Read the model definition and answer for the solid it produces. Units are mm, in the model's axes. Face numbers are marked on the shaded views. A direction names the side the tool comes from. Coordinates: 2 decimals unless noted, no trailing zeros. Order: outer loops, then holes, each group sorted by start corner. A loop starts at its lowest first (then second) coordinate and runs counter-clockwise, first axis right, second up. Notation, with made-up numbers: (59, -2.75) -> (117, -2.75) arc R27 ccw to (117, 14.25) -> close; hole circle Ø5 at (-32, 11.5). An arc over 180 degrees is marked (long way). Answer in a Markdown table with one row per item.
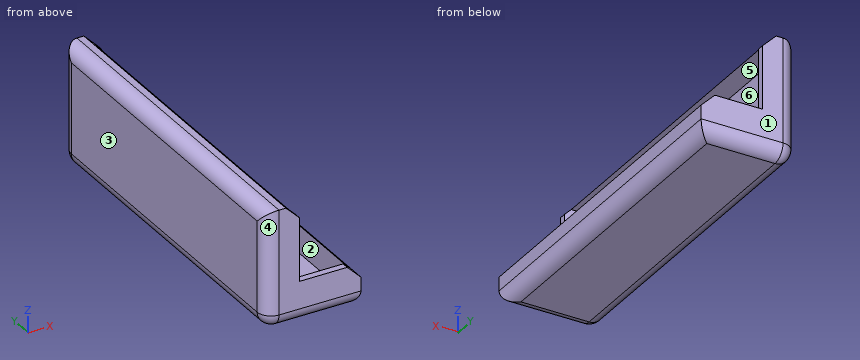
from build123d import *

# Parameters (mm, degrees)
F0_W        = 22.6290904153
F0_H        = 15.2400004526
F1_DEPTH    = 127
F2_T        = -2.54
F3_R        = 5.08
F4_T1_DEPTH = 153.1282991577


# Not quite as in the source:
# - a fillet or chamfer that OpenCascade refuses, or shapes differently, is made with other operations: its cross-section is extruded or revolved along the edge and cut away or added


with BuildPart() as f1:
    # F0 (on Front) → F1 (new body)
    with BuildSketch(Plane.XZ):
        Polygon((-22.6290904153, 0), (-22.6290904153, 15.2400004526), (-22.6290904153, 43.6418191694), (-35.3290904153, 43.6418191694), (-35.3290904153, 0), align=None)
        with Locations((-11.3145452077, 7.6200002263)):
            Rectangle(F0_W, F0_H)
    extrude(amount=F1_DEPTH)

    # F2
    f2_openings = [f1.faces().sort_by_distance(p)[0] for p in [
        (-22.62909, -63.5, 29.44091),
        (-11.314545, -63.5, 15.24),
    ]]
    offset(amount=F2_T, openings=f2_openings)

    # F3
    f3_edges = [f1.edges().sort_by_distance(p)[0] for p in [
        (-35.32909, -63.5, 43.641819),
        (0, -63.5, 0),
        (-35.32909, -63.5, 0),
        (-35.32909, 0, 21.82091),
        (-35.32909, -127, 21.82091),
        (-17.664545, -127, 0),
        (-17.664545, 0, 0),
    ]]
    fillet(f3_edges, radius=F3_R)

    # F4: chamfer of 5.08 on 2 edges, made by hand

    # F4_s2 → F4_t1 (cut)
    with BuildSketch(Plane.XZ.offset(-13.0641495789)):
        Polygon((-27.7090904153, 43.6418191694), (-22.6290904153, 38.5618191694), (-22.6290904153, 43.6418191694), align=None)
        Polygon((-5.08, 15.2400004526), (0, 10.1600004526), (0, 15.2400004526), align=None)
    extrude(amount=F4_T1_DEPTH, mode=Mode.SUBTRACT)


solid = f1.part
Q1. Given pin 1 (1.5 mm diameter, centred on y = -34, z = 31, fed in from +X); pin 2 (3 mm diameter, centred on x = -11.5, y = -1.5, fed in from +Z); pin 3 (0.8 mm diameter, centred on y = -1, z = 28, fed in from +X), each flat-ended and moving along its own axis, determine where each tip first touches the part or whether it passes through.
Outcome:
| item | result |
|---|---|
| pin 1 | x = -32.79 |
| pin 2 | z = 15.24 |
| pin 3 | x = -22.63 |
Q2. The part is cut by section C-C (z = 14). Write down the section's boundary in (x, y).
Outcome:
| item | result |
|---|---|
| outline | (-35.33, -121.92) arc R5.08 ccw to (-30.25, -127) -> (-3.84, -127) -> (-3.84, -124.46) -> (-32.79, -124.46) -> (-32.79, -2.54) -> (-3.84, -2.54) -> (-3.84, 0) -> (-30.25, 0) arc R5.08 ccw to (-35.33, -5.08) -> close |
Q3. The part is cut by section B-B (y = -91). Write down the section's boundary in (x, z).
Outcome:
| item | result |
|---|---|
| outline | (-35.33, 5.08) arc R5.08 ccw to (-30.25, 0) -> (-5.08, 0) arc R5.08 ccw to (0, 5.08) -> (0, 10.16) -> (-2.54, 12.7) -> (-2.54, 2.54) -> (-32.79, 2.54) -> (-32.79, 41.1) -> (-25.17, 41.1) -> (-27.71, 43.64) -> (-30.25, 43.64) arc R5.08 ccw to (-35.33, 38.56) -> close |
Q4. For a pull along X with two mould halves and no side action, classify the marked faces 1, 2 and 3 as pulls with the +X half, pulls with the -X half, needs draft (parallel to the pull), parting line crosses it, or undercut.
Outcome:
| item | result |
|---|---|
| face 1 | needs draft |
| face 2 | undercut |
| face 3 | pulls with the -X half |
Q5. The part is cut by section A-A (x = -8). Write down the section's boundary in (y, z), then the cut area to 3 significant figures.
Outcome:
| item | result |
|---|---|
| outline | (-127, 5.08) arc R5.08 ccw to (-121.92, 0) -> (-5.08, 0) arc R5.08 ccw to (0, 5.08) -> (0, 15.24) -> (-2.54, 15.24) -> (-2.54, 2.54) -> (-124.46, 2.54) -> (-124.46, 15.24) -> (-127, 15.24) -> close |
| area | 376 mm² |
Q6. For the marked faces 4, 5 and 6, determine the directions among +Z, -Z, +X, -X, +Y, -Y from which every point of the face is accessible in a straight line to the end or side of a thin tool.
Outcome:
| item | result |
|---|---|
| face 4 | +Z, -Z, -X, -Y |
| face 5 | +X |
| face 6 | none |
Q7. Consider line 1 (Y direction, x = -26, z = 22); line 2 (Z direction, x = -30, y = -119); line 3 (X direction, y = -98.5, z = 38). Determine where each line is inside the solid, lowest interval first.
Outcome:
| item | result |
|---|---|
| line 1 | -127 to -124.46, -2.54 to 0 |
| line 2 | 0 to 2.54, 41.1 to 43.64 |
| line 3 | -35.33 to -32.79 |
